Source: CAD feature listing. Evaluate the final solid. Frame: model axes, mm. Coordinates: 2 decimals unless noted, no trailing zeros. Order: outer loops, then holes, each group sorted by start corner. A loop starts at its lowest first (then second) coordinate and runs counter-clockwise, first axis right, second up. Notation, with made-up numbers: (75.5, 59) - (83.5, 59) arc R25 ccw to (83.5, 79) - close; hole circle Ø8 at (9.5, -34.5). An arc over 180 degrees is marked (long way). One line per question, with ' | ' between items.
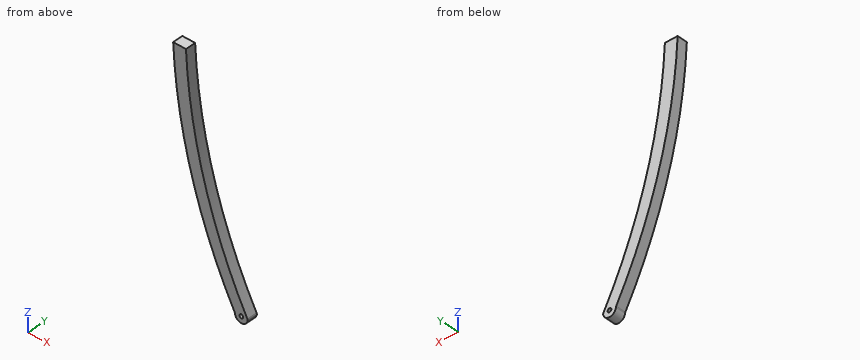
Autodesk Inventor part; units mm, degrees
ref_plane "YZ Plane" through (0, 0, 0) normal (1, 0, 0) x (0, 1, 0)
ref_plane "XZ Plane" through (0, 0, 0) normal (0, 1, 0) x (-1, 0, 0)
ref_plane "XY Plane" through (0, 0, 0) normal (0, 0, 1) x (1, 0, 0)
sketch "Sketch1" plane through (0, 0, 0) normal (0, 1, 0) x (-1, 0, 0)
  line L0 (0, 0) -> (0, -382.775) construction
  line L1 (-5, 0) -> (-5, -382.775)
  line L2 (5, -382.775) -> (5, 0)
  arc A0 (5, 0) -> (-5, 0) centre (0, 0) ccw
  arc A1 (-5, -382.775) -> (5, -382.775) centre (0, -382.775) ccw
  circle A2 centre (0, 0) radius 1.5
  circle A3 centre (0, -382.775) radius 1.5
  arc A4 (5, -382.775) -> (5, 0) centre (-346.2418, -191.3875) ccw
  arc A5 (-5, -382.775) -> (-5, 0) centre (-356.2418, -191.3875) ccw
  point P0 (0, -191.3875)
  dimension "d0" = 382.775
  dimension "d1" = 10
  dimension "d2" = 3
  dimension "d3" = 3
  dimension "d12" = 400
  dimension "d13" = 400
extrude "Extrusion1" add sketch "Sketch1" along normal blind 8 contours A0 L2 A5 | A5 L2 A1 | A4 L2 A5
fillet "Fillet1" radius 2 4 edges at (5, 4, -382.775) (-5, 4, -382.775) (-5, 4, 0) (5, 4, 0)
sketch "Sketch2" plane through (0, 0, 0) normal (0, -1, 0) x (1, 0, 0)
  arc A0 (-4.9846, -383.1668) -> (4.9441, -383.5202) centre (0, -382.775) ccw
  arc A1 (4.9441, 0.7452) -> (-4.9846, 0.3918) centre (0, 0) ccw
  circle A2 centre (0, -382.775) radius 1.5
  circle A3 centre (0, 0) radius 1.5
  arc A4 (-5.2212, -0.4065) -> (-5.2212, -382.3685) centre (346.2418, -191.3875) ccw
  arc A5 (4.7241, -0.5073) -> (4.7241, -382.2677) centre (356.2418, -191.3875) ccw
  arc A6 (4.7241, -0.5073) -> (4.9441, 0.7452) centre (2.9665, 0.4471) ccw
  arc A7 (-5.2212, -0.4065) -> (-4.9846, 0.3918) centre (-6.9785, 0.5485) ccw
  arc A8 (-4.9846, -383.1668) -> (-5.2212, -382.3685) centre (-6.9785, -383.3235) ccw
  arc A9 (4.9441, -383.5202) -> (4.7241, -382.2677) centre (2.9665, -383.2221) ccw
sketch "Sketch3" plane through (0, 8, 0) normal (0, 1, 0) x (1, 0, 0)
  line L0 (-111.727, 425.5197) -> (93.4733, 425.5197)
  line L1 (93.4733, 425.5197) -> (93.4733, -68.38)
  line L2 (93.4733, -68.38) -> (-111.727, -68.38)
  line L3 (-111.727, -68.38) -> (-111.727, 425.5197)
  line L4 (-64.7929, 400.3549) -> (33.9871, 400.3549)
  line L5 (33.9871, 400.3549) -> (33.9871, 210)
  line L6 (33.9871, 210) -> (-64.7929, 210)
  line L7 (-64.7929, 210) -> (-64.7929, 400.3549)
  line L8 (-64.7929, 210) -> (33.9871, 210)
  line L9 (33.9871, 210) -> (33.9871, 30)
  line L10 (33.9871, 30) -> (-64.7929, 30)
  line L11 (-64.7929, 30) -> (-64.7929, 210)
  point P0 (0, 0)
  dimension "d15" = 30
  dimension "d16" = 180
  dimension "d17" = 190.3549
extrude "Extrusion2" cut sketch "Sketch3" along normal mid plane 20 contours L0 L1 L2 L3 | L6 L9 L10 L11
sketch "Sketch4" plane through (0, 8, 0) normal (0, 1, 0) x (1, 0, 0)
  circle A0 centre (0, 382.775) radius 1.5
  line L0 (-53.3249, 210) -> (-43.3249, 210)
  arc A1 (4.7241, 382.2677) -> (-43.3249, 210) centre (356.2418, 191.3875) ccw
  arc A2 (4.7241, 382.2677) -> (4.9441, 383.5202) centre (2.9665, 383.2221) ccw
  arc A3 (4.9441, 383.5202) -> (-4.9846, 383.1668) centre (0, 382.775) ccw
  arc A4 (-5.2212, 382.3685) -> (-4.9846, 383.1668) centre (-6.9785, 383.3235) ccw
  arc A5 (-5.2212, 382.3685) -> (-53.3249, 210) centre (346.2418, 191.3875) ccw
  point P0 (0, 0)
properties part number "Part_13_p1"
(1) Pin query (flat end, axial travel): P1, Ø4, axis at y = 7, z = -302, coming from the +X side; P2, Ø4, axis at x = -2.5, y = 1, coming from the -Z side; P3, Ø2, axis at y = 4, z = -359, coming from the +X side. Return the tip coordinate at first contact, or that it passes through.
Taken from the geometry:
P1: stops at x = -27.58 | P2: stops at z = -387.75 | P3: stops at x = -6.48
(2) Cut plane C-C (z = -374.5). Return the cut outline in (x, y).
Taken from the geometry:
outline: (-9.38, 0) - (0.62, 0) - (0.62, 8) - (-9.38, 8) - close
(3) Cut plane A-A (x = 0). Return the cut outline in (y, z) (3 decimals).
Taken from the geometry:
outline: (0, -387.775) - (8, -387.775) - (8, -384.275) - (0, -384.275) - close; (0, -381.275) - (8, -381.275) - (8, -373.299) - (0, -373.299) - close
(4) Cut plane B-B (x = -29). Return the cut outline in (y, z).
Taken from the geometry:
outline: (0, -329.93) - (8, -329.93) - (8, -299.04) - (0, -299.04) - close
(5) Material intervals for L1, parallel to Z at x = 0, y = 1.5 (3 decimals); L2, parallel to X at y = 6, z = -373.5; L3, parallel to Z at x = -11, y = 5.5, sorted ascending. Write a range as from..to.
Taken from the geometry:
L1: z = -387.775..-384.275, -381.275..-373.299 | L2: x = -9.9..0.1 | L3: z = -371.33..-349.92
